Drawing for the job (mm, zero at the part's lowest x, y, z). A direction names the side the tool comes from. Coordinates: 2 decimals unless noted, no trailing zeros. Write each loop counter-clockwise with the first axis right and the second up, starting at its lowest first coordinate (ties: lowest second). Pieces come first, ordered by that corner, then holes. Notation, with made-up numbers: M -9,81 L 3,81 A23 cw 3,109 Z; hole C 8.5,80 d6. An arc over 180 degrees is marked long. Use a Markdown table: item, result. Add a question column.
Q1. Pin check, flat tips, straight feed: pin 1 Ø3.5 at (x, y) = (5, 4.9) entering from -Z; pin 2 Ø3 at (x, y) = (6.5, 5) entering from -Z; pin 3 Ø1.5 at (x, y) = (8, 1.5) entering from -Z; pin 4 Ø3 at (y, z) = (4, 2.5) entering from -X. Stop position of each tip, or through.
Q2. Wall check: L1, parallel to Y at x = 3, z = 1.5; L2, parallel to Y at x = 5, z = 9.55; L3, parallel to Z at x = 2.75, y = 2.5. Give the ranges that are in metal, low to high. Write a range as from..to.
Q3. Slice it at A-A on z = 7.25. Write the cut outline in (x, y).
Q4. Slice it at B-B on x = 5. Write the cut outline in (y, z), then the cut area to 3 significant figures.
Q5. Slice it at C-C on z = 2.5. Write the cut outline in (x, y).
Q6. Tool access for the marked faces 1 and 2: list every direction of +Z, -Z, +X, -X, +Y, -Y with a clear straight run to the whole face (end or side of a thin tool).
Q7. Mould opens along Z. For the marked faces 3, 4 and 5 say: released by +Z, released by -Z, zero draft, split by the parting line, or undercut.
Q8. Slice it at D-D on x = 9. Write the cut outline in (y, z).
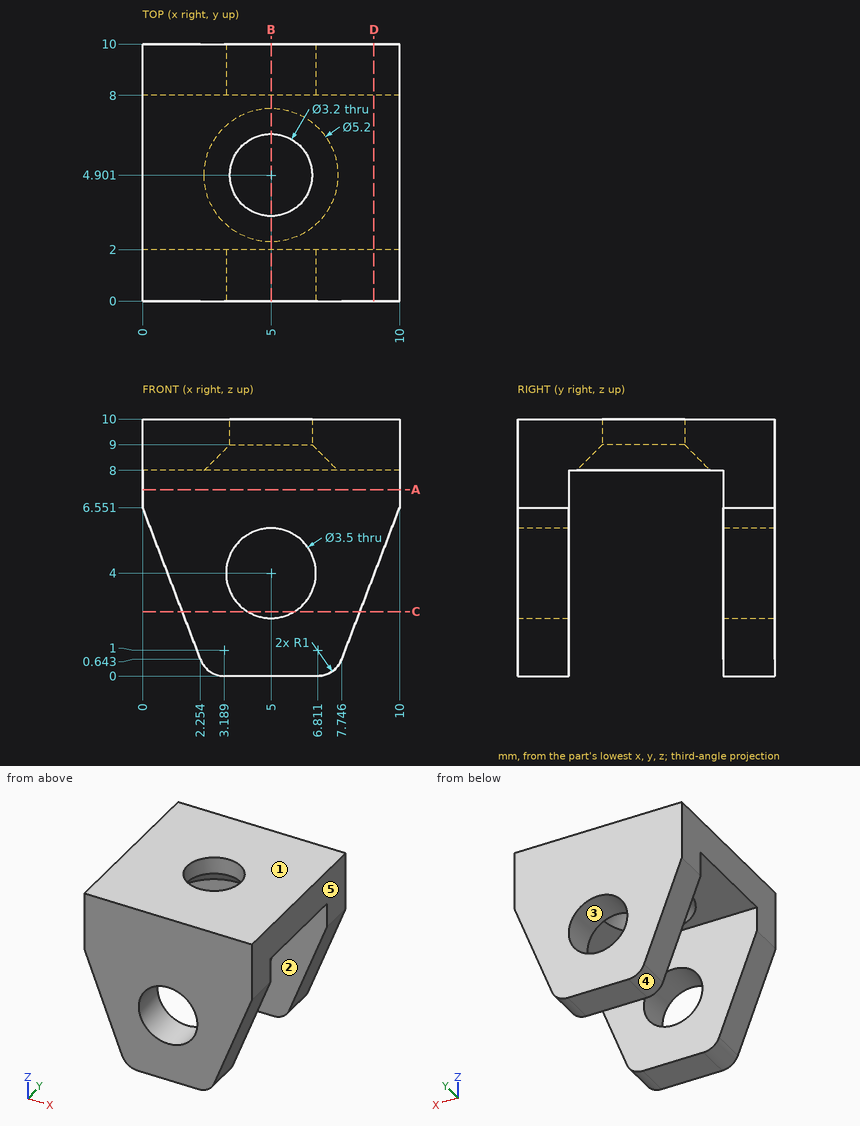
Recorded:
| question | item | result |
|---|---|---|
| 1 | pin 1 | z = 8.85 |
| 1 | pin 2 | z = 8 |
| 1 | pin 3 | z = 0.1 |
| 1 | pin 4 | through |
| 2 | L1 | 0..2, 8..10 |
| 2 | L2 | 0..3.3, 6.5..10 |
| 2 | L3 | 8..10 |
| 3 | outline | M 0,0 L 10,0 L 10,2 L 0,2 Z; M 0,8 L 10,8 L 10,10 L 0,10 Z |
| 4 | outline | M 0,0 L 2,0 L 2,2.25 L 0,2.25 Z; M 0,5.75 L 2,5.75 L 2,8 L 2.3,8 L 3.3,9 L 3.3,10 L 0,10 Z; M 6.5,9 L 7.5,8 L 8,8 L 8,5.75 L 10,5.75 L 10,10 L 6.5,10 Z; M 8,0 L 10,0 L 10,2.25 L 8,2.25 Z |
| 4 | area | 30.6 mm² |
| 5 | outline | M 1.55,0 L 4.1,0 L 4.1,2 L 1.55,2 Z; M 1.55,8 L 4.1,8 L 4.1,10 L 1.55,10 Z; M 5.9,0 L 8.45,0 L 8.45,2 L 5.9,2 Z; M 5.9,8 L 8.45,8 L 8.45,10 L 5.9,10 Z |
| 6 | face 1 | +Z, +X, -X, +Y, -Y |
| 6 | face 2 | -Z, +X, -X |
| 7 | face 3 | undercut |
| 7 | face 4 | released by -Z |
| 7 | face 5 | zero draft |
| 8 | outline | M 0,3.93 L 2,3.93 L 2,8 L 8,8 L 8,3.93 L 10,3.93 L 10,10 L 0,10 Z |
